Read the model definition and answer for the solid it produces. Units are mm, in the model's axes. Face numbers are marked on the shaded views. A direction names the side the tool comes from. Coordinates: 2 decimals unless noted, no trailing zeros. Use one line per item in the form item = value.
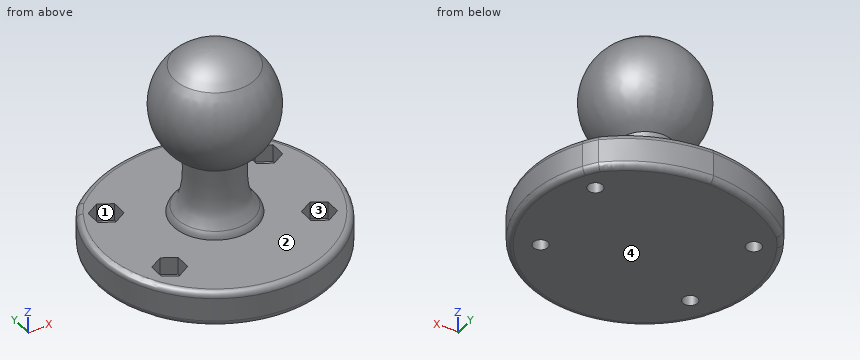
from build123d import *

# Parameters (mm, degrees)
F0_R     = 2.5
F1_DEPTH = 12
F3_R     = 2.5
F4_DEPTH = 6
F5_R     = 2


# Not quite as in the source:
# - a fillet or chamfer that OpenCascade refuses, or shapes differently, is made with other operations: its cross-section is extruded or revolved along the edge and cut away or added


with BuildPart() as f1:
    # F0 (on Top) → F1 (new body)
    with BuildSketch(Plane.XY):
        with BuildLine():
            ThreePointArc((-31.3651592039, 24.7400687451), (-33.0304528025, 22.4689333996), (-34.5318159842, 20.0862527403))
            ThreePointArc((-34.5318159842, 20.0862527403), (0.3556410553, -40.0322385106), (34.289361103, 20.6296959515))
            ThreePointArc((34.289361103, 20.6296959515), (32.9313235996, 22.7293613836), (31.4447447441, 24.7400687451))
            add(Edge.make_bspline(
                [(31.4447447441, 24.7400687451), (22.988602022, 32.1085255021), (13.1297165658, 36.2919575894), (0.0397927701, 36.9132596428)],
                knots=[0, 0, 0, 0, 0.5, 0.5, 0.5, 0.5], degree=3))
            add(Edge.make_bspline(
                [(-31.3651592039, 24.7400687451), (-22.9090164817, 32.1085255021), (-13.0501310255, 36.2919575894), (0.0397927701, 36.9132596428)],
                knots=[0, 0, 0, 0, 0.5, 0.5, 0.5, 0.5], degree=3))
        make_face()
        with Locations((-25.4602072299, -16.0334855318)):
            Circle(F0_R, mode=Mode.SUBTRACT)
        with Locations((25.5397927701, -16.0334855318)):
            Circle(F0_R, mode=Mode.SUBTRACT)
        with Locations((-26.9602072299, 15.9665144682)):
            Circle(F0_R, mode=Mode.SUBTRACT)
        with Locations((27.0397927701, 15.9665144682)):
            Circle(F0_R, mode=Mode.SUBTRACT)
    extrude(amount=F1_DEPTH)

    # F3 (on face) → F4 (cut)
    with BuildSketch(Plane.XY.offset(12)):
        Polygon((-22.4602072299, 13.3684382568), (-22.4602072299, 18.5645906795), (-26.9602072299, 21.1626668909), (-31.4602072299, 18.5645906795), (-31.4602072299, 13.3684382568), (-26.9602072299, 10.7703620455), align=None)
        with Locations((-26.9602072299, 15.9665144682)):
            Circle(F3_R, mode=Mode.SUBTRACT)
        Polygon((22.5397927701, 18.5645906795), (22.5397927701, 13.3684382568), (27.0397927701, 10.7703620455), (31.5397927701, 13.3684382568), (31.5397927701, 18.5645906795), (27.0397927701, 21.1626668909), align=None)
        with Locations((27.0397927701, 15.9665144682)):
            Circle(F3_R, mode=Mode.SUBTRACT)
        Polygon((21.0397927701, -13.4354093205), (21.0397927701, -18.6315617432), (25.5397927701, -21.2296379545), (30.0397927701, -18.6315617432), (30.0397927701, -13.4354093205), (25.5397927701, -10.8373331091), align=None)
        with Locations((25.5397927701, -16.0334855318)):
            Circle(F3_R, mode=Mode.SUBTRACT)
        Polygon((-20.9602072299, -18.6315617432), (-20.9602072299, -13.4354093205), (-25.4602072299, -10.8373331091), (-29.9602072299, -13.4354093205), (-29.9602072299, -18.6315617432), (-25.4602072299, -21.2296379545), align=None)
        with Locations((-25.4602072299, -16.0334855318)):
            Circle(F3_R, mode=Mode.SUBTRACT)
    extrude(amount=-F4_DEPTH, mode=Mode.SUBTRACT)

    # F5
    f5_edges = [f1.edges().sort_by_distance(p)[0] for p in [
        (-2.459557, -39.955325, 12),
        (-2.459557, -39.955325, 0),
        (16.831403, 33.608309, 12),
        (-16.751817, 33.608309, 12),
        (-16.751817, 33.608309, 0),
        (16.831403, 33.608309, 0),
    ]]
    fillet(f5_edges, radius=F5_R)

    # F6 (on Front) → F7 (revolve)
    with BuildSketch(Plane.XZ):
        with BuildLine():
            Line((-14.1540115437, 11.8460487906), (-0.0248217459, 11.8460487906))
            Line((-0.0248217459, 11.8460487906), (-0.0248217459, 12.5021283307))
            Line((-0.0248217459, 12.5021283307), (-0.0248217459, 25.1048319042))
            Line((-0.0248217459, 25.1048319042), (-0.0248217459, 58.8260033315))
            Line((-0.0248217459, 58.8260033315), (-0.0248217459, 64.264058532))
            Line((-0.0248217459, 64.264058532), (-0.0248217459, 69.9135838276))
            ThreePointArc((-0.0248217459, 69.9135838276), (-7.4432934465, 68.4459215755), (-13.744069299, 64.264058532))
            ThreePointArc((-13.744069299, 64.264058532), (-19.3321206406, 47.8233148814), (-9.582830593, 33.4540520906))
            add(Edge.make_bspline(
                [(-14.1540115437, 13.0516188551), (-12.6789047108, 14.5682779679), (-8.9868889419, 18.3642941178), (-9.359245349, 27.7926803584), (-9.582830593, 33.4540520906)],
                knots=[0, 0, 0, 0, 0.3995396892, 1, 1, 1, 1], degree=3))
            Line((-14.1540115437, 13.0516188551), (-14.1540115437, 11.8460487906))
        make_face()
    revolve(axis=Axis((0, 0, 50.5361706018), (0, 0, 1)))

    # F8: fillet of radius 5 on 1 edges, made by hand

    # F8_s1 → F8_t2 (revolve, cut)
    with BuildSketch(Plane.XZ):
        with BuildLine():
            ThreePointArc((-14.1540115437, 12), (-13.716188898, 13.2222804174), (-12.9784286022, 14.2906285974))
            Line((-12.9784286022, 14.2906285974), (-13.0526409195, 14.3576549502))
            ThreePointArc((-13.0526409195, 14.3576549502), (-13.6328295807, 13.7347113697), (-14.2256974002, 13.1213407167))
            Line((-14.2256974002, 13.1213407167), (-14.2540115437, 13.0516188551))
            ThreePointArc((-14.2540115437, 13.0516188551), (-14.2540115437, 12.5258094276), (-14.2517355198, 12.0212137808))
            Line((-14.2517355198, 12.0212137808), (-14.1540115437, 12))
        make_face()
    revolve(axis=Axis((0, 0, 13.0516188551), (0, 0, 1)), mode=Mode.SUBTRACT)


solid = f1.part
Item 1: Each of these flat-tipped pins is pushed along its axis until it touches: P1, Ø4.5, axis at x = -26.5, y = -17.5, coming from the +Z side; P2, Ø10, axis at x = 27, y = 17, coming from the +Z side; P3, Ø2.5, axis at y = 14.5, z = 7.5, coming from the -X side; P4, Ø4, axis at x = 25.54, y = -16.03, coming from the +Z side. Where does it stop, or does it pass through?
Results below:
P1 = 6
P2 = 12
P3 = -37.69
P4 = through
Item 2: For a pull along Y with two mould halves and no side action, classify the marked faces 1 and 2 as +Y half, -Y half, draft (parallel to the pull), parting line (faces both ways), or undercut.
Results below:
face_1 = undercut
face_2 = draft
Item 3: Find the intervals of material crossed by L1, parallel to Z at x = 20, y = 21.5; L2, parallel to Z at x = -15, y = 10.5; L3, parallel to Z at x = -14, y = 6, in increasing order.
Results below:
L1 = 0 to 12
L2 = 0 to 12, 43.71 to 57.16
L3 = 0 to 12, 38.25 to 62.61
Item 4: Which of the six approach directions +Z, -Z, +X, -X, +Y, -Y give full straight-line access (tool end or side, diameter ignored) to the marked faces 3 and 4?
Results below:
face_3 = +Z
face_4 = -Z, +X, -X, +Y, -Y
